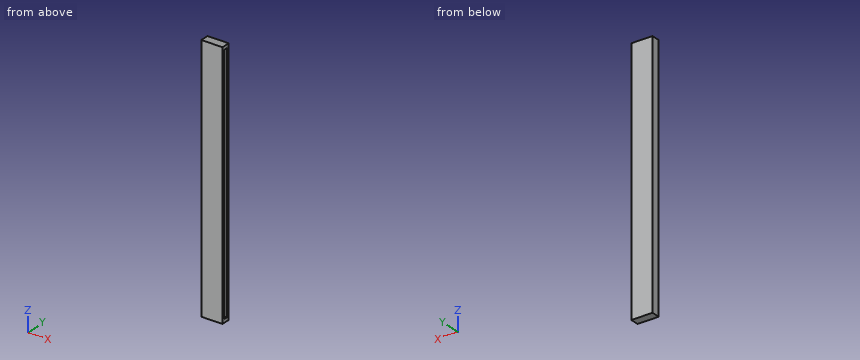
```python
from build123d import *

# Parameters (mm, degrees)
SKETCH_1_W      = 15
SKETCH_1_H      = 300
EXTRUDE_1_DEPTH = 4
SKETCH_2_W      = 4
SKETCH_2_H      = 4
EXTRUDE_2_DEPTH = 10
SKETCH_3_W      = 25
SKETCH_3_H      = 300
EXTRUDE_3_DEPTH = 3
SKETCH_4_W      = 25
SKETCH_4_H      = 300
EXTRUDE_4_DEPTH = 3


with BuildPart() as part:
    # 草图1 → 凸台-拉伸1 (new body)
    with BuildSketch(Plane(origin=(0, 0, 0), x_dir=(1, 0, 0), z_dir=(0, 1, 0))):
        with Locations((-54.836215811, -65.70889057)):
            Rectangle(SKETCH_1_W, SKETCH_1_H)
    extrude(amount=EXTRUDE_1_DEPTH)

    # 草图2 → 凸台-拉伸2 (add)
    with BuildSketch(Plane(origin=(-47.336215811, 0, 0), x_dir=(0, 0, -1), z_dir=(1, 0, 0))):
        with Locations((-213.70889057, 2)):
            Rectangle(SKETCH_2_W, SKETCH_2_H)
        with Locations((82.29110943, 2)):
            Rectangle(SKETCH_2_W, SKETCH_2_H)
    extrude(amount=EXTRUDE_2_DEPTH)

    # 草图3 → 凸台-拉伸3 (add)
    with BuildSketch(Plane(origin=(0, 4, 0), x_dir=(1, 0, 0), z_dir=(0, 1, 0))):
        with Locations((-49.836215811, -65.70889057)):
            Rectangle(SKETCH_3_W, SKETCH_3_H)
    extrude(amount=EXTRUDE_3_DEPTH)

    # 草图4 → 凸台-拉伸4 (add)
    with BuildSketch(Plane.XZ):
        with Locations((-49.836215811, 65.70889057)):
            Rectangle(SKETCH_4_W, SKETCH_4_H)
    extrude(amount=EXTRUDE_4_DEPTH)


solid = part.part
```
CAD build for the part. Positions are in the model's coordinates, mm. Round coordinates to 2 decimals unless told otherwise and drop trailing zeros. Order: outer loops, then holes, each group sorted by start corner. A loop starts at its lowest first (then second) coordinate and runs counter-clockwise, first axis right, second up.
Q1. Slice it at C-C (z = 6). Write the cut outline in (x, y).
Q2. Slice it at B-B (y = 2.25). Write the cut outline in (x, z).
Q3. Slice it at A-A (x = -41.5). Write the cut outline in (y, z).
Q4. Wall check: L1, parallel to Z at x = -47, y = 2; L2, parallel to Y at x = -38.5, z = 197.5; L3, parallel to X at y = 1.5, z = 159.5. Give the ranges that are in metal, low to high.
Results below:
1. outline: (-62.34, -3) - (-37.34, -3) - (-37.34, 0) - (-47.34, 0) - (-47.34, 4) - (-37.34, 4) - (-37.34, 7) - (-62.34, 7) - close
2. outline: (-62.34, -84.29) - (-37.34, -84.29) - (-37.34, -80.29) - (-47.34, -80.29) - (-47.34, 211.71) - (-37.34, 211.71) - (-37.34, 215.71) - (-62.34, 215.71) - close
3. outline: (-3, -84.29) - (7, -84.29) - (7, 215.71) - (-3, 215.71) - close; hole (0, -80.29) - (4, -80.29) - (4, 211.71) - (0, 211.71) - close
4. L1: z = -84.29 to -80.29, 211.71 to 215.71
4. L2: y = -3 to 0, 4 to 7
4. L3: x = -62.34 to -47.34
